```python
from build123d import *

# Parameters (mm, degrees)
SKETCH_1_W                     = 108
SKETCH_1_H                     = 11
EXTRUDE_1_DEPTH                = 7.5
CUT_EXTRUDE_1_DEPTH            = 16
FILLET_1_R                     = 0.76
PATTERN_LINEAR_1_COUNT         = 17
PATTERN_LINEAR_1_PITCH         = 6.28
FILLET_1_OF_PATTERN_LINEAR_1_R = 0.76
SKETCH_3_W                     = 15
SKETCH_3_H                     = 11
EXTRUDE_2_DEPTH                = 44.58
SKETCH_4_W                     = 15
SKETCH_4_H                     = 11
CUT_EXTRUDE_2_DEPTH            = 33.02
SKETCH_5_R                     = 2.5
CUT_EXTRUDE_3_DEPTH            = 10


with BuildPart() as part:
    # 草图1 → 凸台-拉伸1 (new body, symmetric)
    with BuildSketch(Plane.XY):
        Rectangle(SKETCH_1_W, SKETCH_1_H)
    extrude(amount=EXTRUDE_1_DEPTH, both=True)

    # 草图2 → 切除-拉伸1 (cut, through all)
    with BuildSketch(Plane.XY.offset(7.5)):
        Polygon((-52.43, 5.5), (-47.834119063, 5.5), (-49.471985117, 1), (-50.792133946, 1), align=None)
    cut_extrude_1 = extrude(amount=-CUT_EXTRUDE_1_DEPTH, mode=Mode.SUBTRACT)

    # 圆角1
    fillet_1_edges = [part.edges().sort_by_distance(p)[0] for p in [
        (-50.792133946, 1, 0),
        (-52.43, 5.5, 0),
        (-47.834119063, 5.5, 0),
        (-49.471985117, 1, 0),
    ]]
    fillet(fillet_1_edges, radius=FILLET_1_R)

    # 阵列(线性)1: 切除-拉伸1 ×17
    with Locations(*[(i * PATTERN_LINEAR_1_PITCH, 0, 0) for i in range(1, PATTERN_LINEAR_1_COUNT)]):
        add(cut_extrude_1, mode=Mode.SUBTRACT)

    # 圆角1 of 阵列(线性)1
    fillet_1_of_pattern_linear_1_edges = [part.edges().sort_by_distance(p)[0] for p in [
        (-44.512133946, 1, 0),
        (-46.15, 5.5, 0),
        (-41.554119063, 5.5, 0),
        (-43.191985117, 1, 0),
        (-38.232133946, 1, 0),
        (-39.87, 5.5, 0),
        (-35.274119063, 5.5, 0),
        (-36.911985117, 1, 0),
        (-31.952133946, 1, 0),
        (-33.59, 5.5, 0),
        (-28.994119063, 5.5, 0),
        (-30.631985117, 1, 0),
        (-25.672133946, 1, 0),
        (-27.31, 5.5, 0),
        (-22.714119063, 5.5, 0),
        (-24.351985117, 1, 0),
        (-19.392133946, 1, 0),
        (-21.03, 5.5, 0),
        (-16.434119063, 5.5, 0),
        (-18.071985117, 1, 0),
        (-13.112133946, 1, 0),
        (-14.75, 5.5, 0),
        (-10.154119063, 5.5, 0),
        (-11.791985117, 1, 0),
        (-6.832133946, 1, 0),
        (-8.47, 5.5, 0),
        (-3.874119063, 5.5, 0),
        (-5.511985117, 1, 0),
        (-0.552133946, 1, 0),
        (-2.19, 5.5, 0),
        (2.405880937, 5.5, 0),
        (0.768014883, 1, 0),
        (5.727866054, 1, 0),
        (4.09, 5.5, 0),
        (8.685880937, 5.5, 0),
        (7.048014883, 1, 0),
        (12.007866054, 1, 0),
        (10.37, 5.5, 0),
        (14.965880937, 5.5, 0),
        (13.328014883, 1, 0),
        (18.287866054, 1, 0),
        (16.65, 5.5, 0),
        (21.245880937, 5.5, 0),
        (19.608014883, 1, 0),
        (24.567866054, 1, 0),
        (22.93, 5.5, 0),
        (27.525880937, 5.5, 0),
        (25.888014883, 1, 0),
        (30.847866054, 1, 0),
        (29.21, 5.5, 0),
        (33.805880937, 5.5, 0),
        (32.168014883, 1, 0),
        (37.127866054, 1, 0),
        (35.49, 5.5, 0),
        (40.085880937, 5.5, 0),
        (38.448014883, 1, 0),
        (43.407866054, 1, 0),
        (41.77, 5.5, 0),
        (46.365880937, 5.5, 0),
        (44.728014883, 1, 0),
        (49.687866054, 1, 0),
        (48.05, 5.5, 0),
        (52.645880937, 5.5, 0),
        (51.008014883, 1, 0),
    ]]
    fillet(fillet_1_of_pattern_linear_1_edges, radius=FILLET_1_OF_PATTERN_LINEAR_1_R)

    # 草图3 → 凸台-拉伸2 (add)
    with BuildSketch(Plane(origin=(9.42, 0, 0), x_dir=(0, 0, -1), z_dir=(1, 0, 0))):
        Rectangle(SKETCH_3_W, SKETCH_3_H)
    extrude(amount=EXTRUDE_2_DEPTH)

    # 草图4 → 切除-拉伸2 (cut, through all)
    with BuildSketch(Plane(origin=(21.98, 0, 0), x_dir=(0, 0, -1), z_dir=(1, 0, 0))):
        Rectangle(SKETCH_4_W, SKETCH_4_H)
    extrude(amount=CUT_EXTRUDE_2_DEPTH, mode=Mode.SUBTRACT)

    # 草图5 → 切除-拉伸3 (cut)
    with BuildSketch(Plane(origin=(21.98, 0, 0), x_dir=(0, 0, -1), z_dir=(1, 0, 0))):
        Circle(SKETCH_5_R)
    extrude(amount=-CUT_EXTRUDE_3_DEPTH, mode=Mode.SUBTRACT)


solid = part.part
```
Build history of the part. All positions in model axes, mm. A direction names the side the tool comes from. Give positions to 0.01 mm unless a question says otherwise; leave off trailing zeros. Order: outer loops, then holes, each group sorted by start corner. A loop starts at its lowest first (then second) coordinate and runs counter-clockwise, first axis right, second up. Notation, with made-up numbers: M 60,67.5 L 79,67.5 A11 cw 79,76.5 Z; hole C -2.5,-25.5 d8. An arc over 180 degrees is marked long. Return JSON: item names as keys, results as strings.
Q1. 3-axis set-ups, long thin cutter, end or side, ignore diameter. For faces 1 (the face through (-17, -5.5, 0)), 2 (the face through (-17.244, 3.274, 0.105)): which of +Z, -Z, +X, -X, +Y, -Y reach the whole face in a straight line?
Answer list:
{"face 1": "+Z, -Z, +X, -X, -Y", "face 2": "+Z, -Z, +Y"}
Q2. Flat gauge pins, fed straight in: pin 1 (3 mm diameter, centred on x = 1, z = -5.5, fed in from +Y); pin 2 (2.5 mm diameter, centred on y = -1, z = 0, fed in from +X); pin 3 (3 mm diameter, centred on x = 5.5, y = 2.5, fed in from -Z). Where does each tip first touch, or does it go through?
Answer list:
{"pin 1": "stops at y = 5.36", "pin 2": "stops at x = 11.98", "pin 3": "stops at z = -7.5"}
Q3. Band-saw the part on A-A (y = 0). Give the cut face in (x, z).
Answer list:
{"outline": "M -54,-7.5 L 21.98,-7.5 L 21.98,-2.5 L 11.98,-2.5 L 11.98,2.5 L 21.98,2.5 L 21.98,7.5 L -54,7.5 Z"}
Q4. Band-saw the part on B-B (y = 3.25). Count the separate pieces of the cut face and the enclosed holes in it, then the cut area to 3 significant figures.
Answer list:
{"separate pieces": "11", "enclosed holes": "0", "area": "696 mm^2"}
Q5. Wall check: probe 1 along Y at (x, z) = (18.25, 0); probe 2 along Y at (x, z) = (-44, -3.5); probe 3 along Y at (x, z) = (13, -0.5). Give the ranges that are in metal, low to high. Write a range as from..to.
Answer list:
{"probe 1": "y = -5.5..-2.5, 2.5..5.5", "probe 2": "y = -5.5..1", "probe 3": "y = -5.5..-2.45, 2.45..5.5"}
Q6. Two-plate mould, pull along X, no slides. Class faces 3 (the face through (-17, -1, -7.5)), 4 (the face through (-20.202, 3.226, 0.105)), 5 (the face through (-54, 0, 0)): pulls with the +X half, pulls with the -X half, needs draft (parallel to the pull), parting line crosses it, or undercut.
Answer list:
{"face 3": "needs draft", "face 4": "undercut", "face 5": "pulls with the -X half"}
